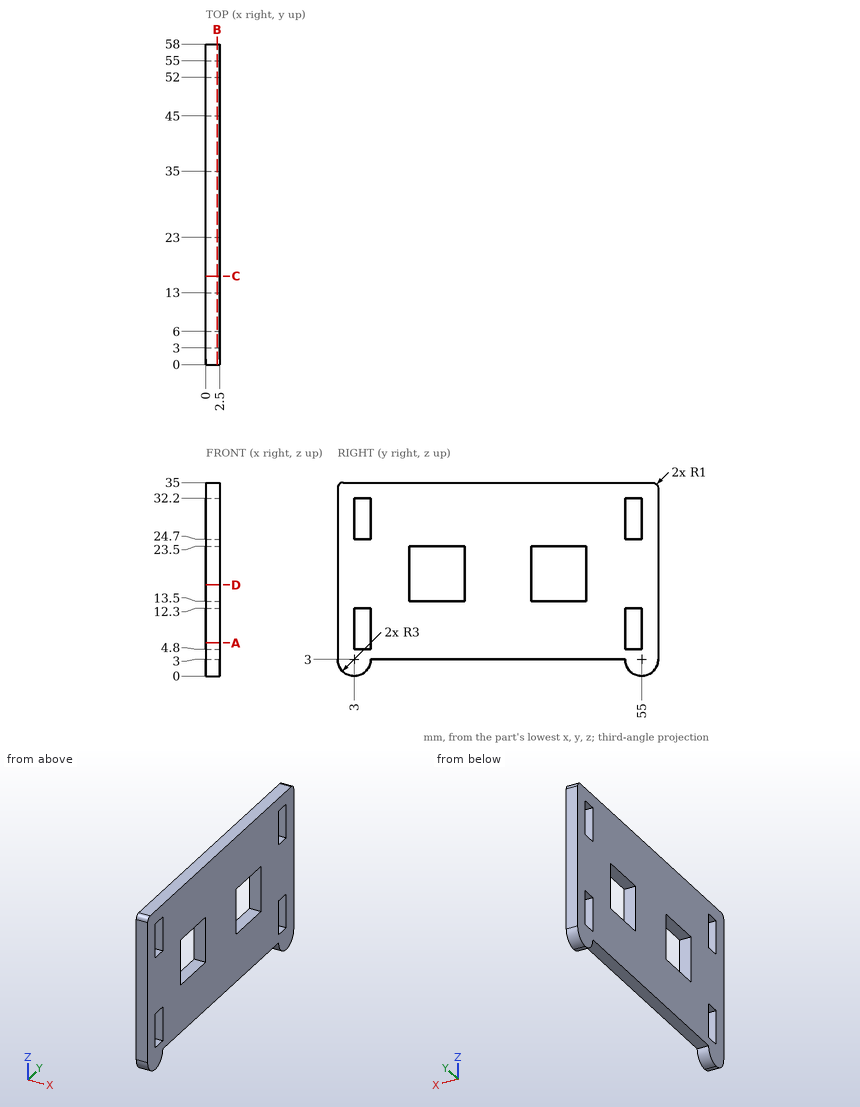
Can you work these out from the drawing? Everything is in mm from the part's minimum corner. Give positions to 0.01 mm unless a question says otherwise; leave off trailing zeros. Order: outer loops, then holes, each group sorted by start corner. A loop starts at its lowest first (then second) coordinate and runs counter-clockwise, first axis right, second up. Notation, with made-up numbers: M -6,0 L 50,0 A15 ccw 50,25 Z; hole C -18.75,7 d8. An arc over 180 degrees is marked long. One line per question, with ' | ' between items.
1. If I drill on line 1 (Y direction, x = 1.15, z = 11); line 2 (Y direction, x = 0.1, z = 19); line 3 (Z direction, x = 1.9, y = 52.5), over which ranges is the centre line in solid material (lowest first)?
Results:
line 1: 0 to 3, 6 to 52, 55 to 58 | line 2: 0 to 13, 23 to 35, 45 to 58 | line 3: 1.34 to 4.8, 12.3 to 24.7, 32.2 to 35
2. I want a section at D-D (z = 16.5). List the corners of the cut face in (x, y) for me, and give its area (3 significant figures).
Results:
outline: M 0,0 L 2.5,0 L 2.5,13 L 0,13 Z; M 0,23 L 2.5,23 L 2.5,35 L 0,35 Z; M 0,45 L 2.5,45 L 2.5,58 L 0,58 Z | area: 95.0 mm²
3. I'm going to push a flat-ended pin straight in: pin 1 (0.8 mm diameter, centred on x = 1, y = 30.5, fed in from -Z). Where does the tip first touch, or does it pass through?
Results:
pin 1: z = 3
4. I want a section at B-B (x = 2.05). Give the number of separate pieces and of enclosed holes in the cut face, and give its area (3 significant figures).
Results:
separate pieces: 1 | enclosed holes: 6 | area: 1,590 mm²
5. I want a section at C-C (y = 16). List the corners of the cut face in (x, z) for me, and give its area (3 significant figures).
Results:
outline: M 0,3 L 2.5,3 L 2.5,13.5 L 0,13.5 Z; M 0,23.5 L 2.5,23.5 L 2.5,35 L 0,35 Z | area: 55.0 mm²
6. I want a section at A-A (z = 6). List the corners of the cut face in (x, y) for me, and give its area (3 significant figures).
Results:
outline: M 0,0 L 2.5,0 L 2.5,3 L 0,3 Z; M 0,6 L 2.5,6 L 2.5,52 L 0,52 Z; M 0,55 L 2.5,55 L 2.5,58 L 0,58 Z | area: 130 mm²
